Geometry: final body of the model. Coordinates: model frame, mm. A direction names the side the tool comes from. Give positions to 0.01 mm unless a question says otherwise; leave off trailing zeros. Order: outer loops, then holes, each group sorted by start corner. A loop starts at its lowest first (then second) coordinate and runs counter-clockwise, first axis right, second up. Notation, with made-up numbers: (76, -37) - (110, -37) arc R19 ccw to (110, -8) - close; hole circle Ø1 at (-40, 87). An arc over 180 degrees is marked (long way). One line per item, written item: value.
```python
from build123d import *

# Parameters (mm, degrees)
F0_R     = 4.7625
F1_DEPTH = 12.7
F2_START = 1.5875
F0_R_2   = 2.1844
F2_DEPTH = 11.1125
F3_START = 1.5875
F3_DEPTH = 11.1125


# Not quite as in the source:
# - a feature names something its author has since deleted; it is built from what else it names


with BuildPart() as f1:
    # F0 (on Front) → F1 (new body)
    with BuildSketch(Plane.XZ):
        Polygon((97.3731166124, 28.1938837487), (97.3731166124, 34.5438837487), (-140.7518833876, 34.5438837487), (-140.7518833876, 28.5026916087), (-134.4018833876, 28.5026916087), (-134.4018833876, 22.1526916087), (-140.7518833876, 22.1526916087), (-140.7518833876, 15.8026916087), (-134.4018833876, 15.8026916087), (-134.4018833876, 9.4526916087), (-140.7518833876, 9.4526916087), (-140.7518833876, 3.7844837487), (-134.4018833876, 3.7844837487), (-134.4018833876, -3.2473083913), (-140.7518833876, -3.2473083913), (-140.7518833876, -9.5973083913), (-134.4018833876, -9.5973083913), (-134.4018833876, -15.9473083913), (-140.7518833876, -15.9473083913), (-140.7518833876, -22.6061162513), (-115.3518833876, -22.6061162513), (-115.3518833876, -16.2561162513), (-96.3018833876, -16.2561162513), (-96.3018833876, -22.6061162513), (-73.2831333876, -22.6061162513), (-73.2831333876, -16.2561162513), (-54.2331333876, -16.2561162513), (-54.2331333876, -22.6061162513), (-31.2143833876, -22.6061162513), (-31.2143833876, -16.2561162513), (-12.1643833876, -16.2561162513), (-12.1643833876, -22.6061162513), (10.8543666124, -22.6061162513), (10.8543666124, -16.2561162513), (29.9043666124, -16.2561162513), (29.9043666124, -22.6061162513), (52.9231166124, -22.6061162513), (52.9231166124, -16.2561162513), (71.9731166124, -16.2561162513), (71.9731166124, -22.6061162513), (97.3731166124, -22.6061162513), (97.3731166124, -16.2561162513), (91.0231166124, -16.2561162513), (91.0231166124, -9.9061162513), (97.3731166124, -9.9061162513), (97.3731166124, -3.5561162513), (91.0231166124, -3.5561162513), (91.0231166124, 2.7938837487), (97.3731166124, 2.7938837487), (97.3731166124, 9.1438837487), (91.0231166124, 9.1438837487), (91.0231166124, 15.4938837487), (97.3731166124, 15.4938837487), (97.3731166124, 21.8438837487), (91.0231166124, 21.8438837487), (91.0231166124, 28.1938837487), align=None)
        with Locations((-53.4393833876, 5.9688837487)):
            Circle(F0_R, mode=Mode.SUBTRACT)
        with Locations((10.0606166124, 5.9688837487)):
            Circle(F0_R, mode=Mode.SUBTRACT)
    extrude(amount=F1_DEPTH)

    # F0 (on Front) → F2 (join)
    with BuildSketch(Plane.XZ.offset(F2_START)):
        with Locations((-53.4393833876, 5.9688837487)):
            Circle(F0_R)
        with Locations((-53.4393833876, 5.9688837487)):
            Circle(F0_R_2, mode=Mode.SUBTRACT)
    extrude(amount=F2_DEPTH)

    # F0 (on Front) → F3 (join)
    with BuildSketch(Plane.XZ.offset(F3_START)):
        with Locations((10.0606166124, 5.9688837487)):
            Circle(F0_R)
        with Locations((10.0606166124, 5.9688837487)):
            Circle(F0_R_2, mode=Mode.SUBTRACT)
    extrude(amount=F3_DEPTH)


solid = f1.part
```
1) Material intervals for line 1 along X through (y, z) = (-4.5, 7.5); line 2 along Z through (x, y) = (-26, -7); line 3 along X through (y, z) = (-5.75, 27), sorted ascending.
Answers below:
line 1: -140.75 to -55, -51.88 to 8.5, 11.62 to 97.37
line 2: -16.26 to 34.54
line 3: -134.4 to 91.02
2) Mould query, pull axis X, two halves, no side actions, for faces 1 (the face through (-140.752, -6, 7)), 2 (the face through (-138, -6, 9.453)), 3 (the face through (10.854, -6, -19)), 4 (the face through (29.904, -6, -19)). Classes: released by +X, released by -X, zero draft, split by the parting line, or undercut.
Answers below:
face 1: released by -X
face 2: zero draft
face 3: undercut
face 4: undercut
3) Set-up query: faces 5 (the face through (-134.402, -6, -13)), 6 (the face through (71.973, -6, -19)), 7 (the face through (-140.752, -6, -19)), 8 (the face through (94, -6, -3.556)). Return all of +Z, -Z, +X, -X, +Y, -Y with unobstructed straight access to the full face (end or side cutting, diameter ignored); none if empty.
Answers below:
face 5: -X, +Y, -Y
face 6: -Z, +Y, -Y
face 7: +Z, -Z, -X, +Y, -Y
face 8: +X, +Y, -Y
4) Section A-A, the plane x = 65. Return loops of the section in (y, z), then the cut area to 3 significant figures.
Answers below:
outline: (-12.7, -16.26) - (0, -16.26) - (0, 34.54) - (-12.7, 34.54) - close
area: 645 mm^2
5) Section B-B, the plane y = -8.5. Count the separate pieces of the cut face and the enclosed holes in it, then the cut area to 3 significant figures.
Answers below:
separate pieces: 1
enclosed holes: 2
area: 12,600 mm^2
6) First-contact query: pin 1 (3 mm diameter, centred on x = -102, y = -8.5, fed in from -Z); pin 2 (7 mm diameter, centred on y = -6, z = 10.5, fed in from +X); pin 3 (3 mm diameter, centred on y = -5, z = -0.5, fed in from +X). Flat tips, straight axial feed; report the tip coordinate or a pass-through.
Answers below:
pin 1: z = -16.26
pin 2: x = 97.37
pin 3: x = 91.02
